Verification items for the finished model (mm, model axes). A direction names the side the tool comes from. Coordinates: 2 decimals unless noted, no trailing zeros. Write each loop counter-clockwise with the first axis right and the second up, starting at its lowest first coordinate (ties: lowest second). Pieces come first, ordered by that corner, then holes.
```python
from build123d import *

# Parameters (mm, degrees)
EXTRUDE_1_DEPTH     = 5.5
EXTRUDE_2_DEPTH     = 1
SKETCH_3_R          = 2
CUT_EXTRUDE_1_DEPTH = 0.5
FILLET_1_R          = 1


with BuildPart() as part:
    # 草图1 → 凸台-拉伸1 (new body)
    with BuildSketch(Plane.XY):
        with BuildLine():
            Line((2.3, -2.3), (-2.3, -2.3))
            ThreePointArc((-2.3, -2.3), (-4.6, 0), (-2.3, 2.3))
            Line((-2.3, 2.3), (2.3, 2.3))
            ThreePointArc((2.3, 2.3), (4.6, 0), (2.3, -2.3))
        make_face()
    extrude(amount=EXTRUDE_1_DEPTH)

    # 草图2 → 凸台-拉伸2 (add)
    with BuildSketch(Plane(origin=(0, 0, 0), x_dir=(-1, 0, 0), z_dir=(0, 0, -1))):
        with BuildLine():
            Line((2.8, -2.8), (-2.3, -2.8))
            ThreePointArc((-2.3, -2.8), (-2.653553391, -2.653553391), (-2.8, -2.3))
            Line((-2.8, -2.3), (-2.8, 2.3))
            ThreePointArc((-2.8, 2.3), (-2.653553391, 2.653553391), (-2.3, 2.8))
            Line((-2.3, 2.8), (2.8, 2.8))
            ThreePointArc((2.8, 2.8), (5.6, 0), (2.8, -2.8))
        make_face()
    extrude(amount=-EXTRUDE_2_DEPTH)

    # 草图3 → 切除-拉伸1 (cut)
    with BuildSketch(Plane(origin=(0, 0, 0), x_dir=(-1, 0, 0), z_dir=(0, 0, -1))):
        Circle(SKETCH_3_R)
    extrude(amount=-CUT_EXTRUDE_1_DEPTH, mode=Mode.SUBTRACT)

    # 圆角1
    fillet_1_edges = [part.edges().sort_by_distance(p)[0] for p in [
        (-4.6, 0, 5.5),
        (0, -2.3, 5.5),
        (4.6, 0, 5.5),
        (0, 2.3, 5.5),
    ]]
    fillet(fillet_1_edges, radius=FILLET_1_R)


solid = part.part
```
1. Sectioned sample at A-A, the plane y = 0. Record the boundary of the cut face in (x, z).
2. Sectioned sample at C-C, the plane z = 1.3. Record the boundary of the cut face in (x, y).
3. Gauge pin test, flat ends, axial feed: P1, Ø3, axis at x = 3.5, z = 2.5, coming from the +Y side; P2, Ø1, axis at x = -4, y = 2, coming from the +Z side; P3, Ø1, axis at y = 1, z = 3, coming from the +X side (3 decimals). Record the tip position at first contact, or that the pin passes through.
4. Sectioned sample at D-D, the plane x = -1.75. Record the boundary of the cut face in (y, z), and give its area (3 significant figures).
5. Tool access check on faces 1 (the flat face through (0, 2.3, 3)), 2 (the flat face through (0, 0, 0.5)), 3 (the cylindrical face through (-4.6, -0.05, 2.73)), 4 (the flat face through (0, -2.3, 3)). Record the directions out of +Z, -Z, +X, -X, +Y, -Y that give a thin tool (end or side, any length) a straight path to the whole face; none if there is none.
6. Sectioned sample at B-B, the plane x = 0. Record the boundary of the cut face in (y, z), and give its area (3 significant figures).
7. Draft check along Y on faces 5 (the flat face through (-5, 1, 1)), 6 (the cylindrical face through (-0.032, -2.015, 5.199)), 7 (the cylindrical face through (0.434, -1.952, 0.246)), 8 (the cylindrical face through (4.6, 0.05, 2.22)). Enter one of: pulls with the +Y half, pulls with the -Y half, needs draft (parallel to the pull), parting line crosses it, or undercut.
8. Material ranges on L1, parallel to Y at x = 0, z = 0.2; L2, parallel to Z at x = -1.5, y = 1.2; L3, parallel to Y at x = -1.5, z = 1.25, recorded low to high.
Outcome:
1. outline: (-5.6, 0) - (-2, 0) - (-2, 0.5) - (2, 0.5) - (2, 0) - (4.6, 0) - (4.6, 4.5) arc R1 ccw to (3.6, 5.5) - (-3.6, 5.5) arc R1 ccw to (-4.6, 4.5) - (-4.6, 1) - (-5.6, 1) - close
2. outline: (-2.3, -2.3) - (2.3, -2.3) arc R2.3 ccw to (2.3, 2.3) - (-2.3, 2.3) arc R2.3 ccw to start
3. P1: stops at y = 2.3
3. P2: stops at z = 5.07
3. P3: stops at x = 4.545
4. outline: (-2.8, 0) - (-0.97, 0) - (-0.97, 0.5) - (0.97, 0.5) - (0.97, 0) - (2.8, 0) - (2.8, 1) - (2.3, 1) - (2.3, 4.5) arc R1 ccw to (1.3, 5.5) - (-1.3, 5.5) arc R1 ccw to (-2.3, 4.5) - (-2.3, 1) - (-2.8, 1) - close
4. area: 24.9 mm2
5. face 1: +Z, +X, -X, +Y
5. face 2: -Z
5. face 3: +Z, -X
5. face 4: +Z, +X, -X, -Y
6. outline: (-2.8, 0) - (-2, 0) - (-2, 0.5) - (2, 0.5) - (2, 0) - (2.8, 0) - (2.8, 1) - (2.3, 1) - (2.3, 4.5) arc R1 ccw to (1.3, 5.5) - (-1.3, 5.5) arc R1 ccw to (-2.3, 4.5) - (-2.3, 1) - (-2.8, 1) - close
6. area: 23.9 mm2
7. face 5: needs draft
7. face 6: pulls with the -Y half
7. face 7: undercut
7. face 8: parting line crosses it
8. L1: y = -2.8 to -2, 2 to 2.8
8. L2: z = 0.5 to 5.5
8. L3: y = -2.3 to 2.3
